Check sheet for the drawn part. Datum: minimum x, y, z corner. Units: mm. A direction names the side the tool comes from. Round coordinates to 2 decimals unless told otherwise and drop trailing zeros. Write each loop counter-clockwise with the first axis right and the second up, starting at its lowest first coordinate (ties: lowest second). Pieces come first, ordered by that corner, then holes. Notation, with made-up numbers: (65, -11) - (113, -11) arc R21 ccw to (113, 18) - close; hole circle Ø6 at (1, 84.25). An arc over 180 degrees is marked (long way). Answer as a JSON object with one key per item and string values.
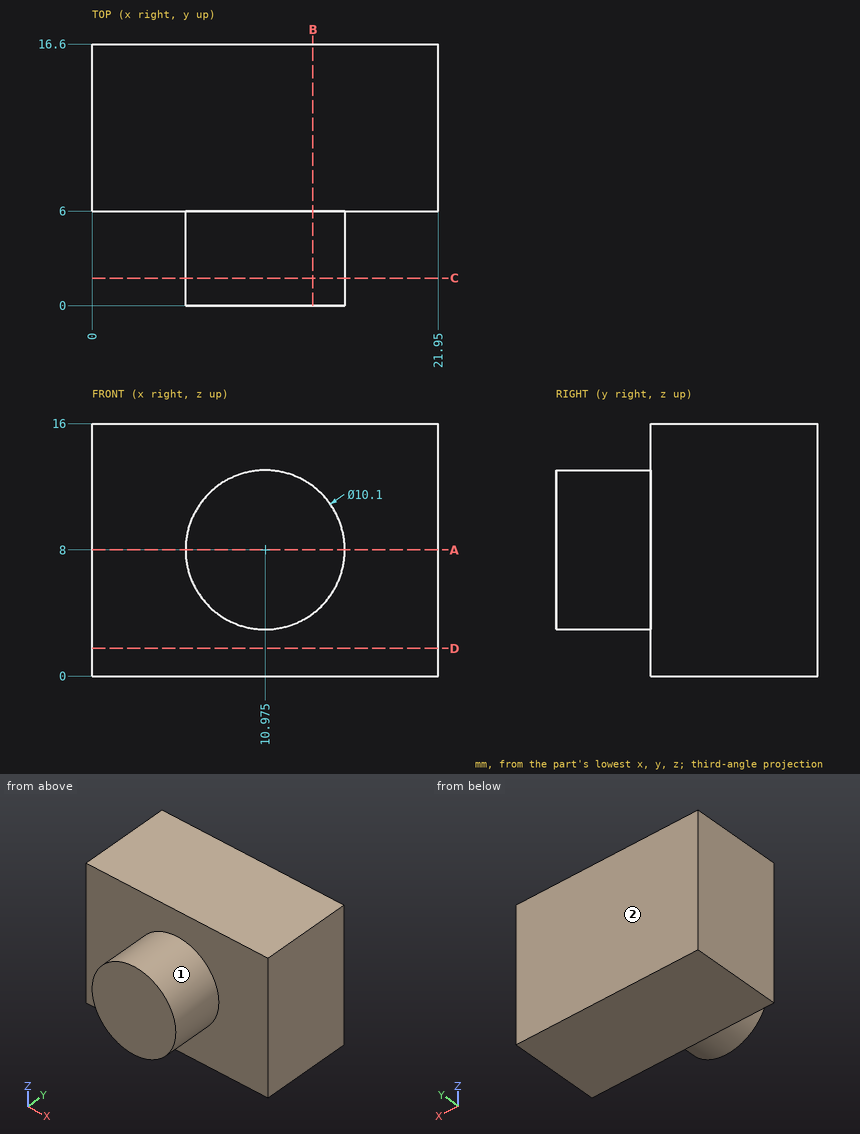
Q1. Section check D-D, the plane z = 1.75. Record the cut outline in (x, y).
Geometry check:
{"outline": "(0, 6) - (21.95, 6) - (21.95, 16.6) - (0, 16.6) - close"}
Q2. Set-up check for the marked faces 1 and 2: record each of +Z, -Z, +X, -X, +Y, -Y from which the full face is reachable in a straight line by a thin tool's end or side.
Geometry check:
{"face 1": "-Y", "face 2": "+Z, -Z, +X, -X, +Y"}
Q3. Section check B-B, the plane x = 14. Record the cut outline in (y, z).
Geometry check:
{"outline": "(0, 3.96) - (6, 3.96) - (6, 0) - (16.6, 0) - (16.6, 16) - (6, 16) - (6, 12.04) - (0, 12.04) - close"}
Q4. Section check C-C, the plane y = 1.75. Record the cut outline in (x, z) (3 decimals).
Geometry check:
{"outline": "circle Ø10.1 at (10.975, 8)"}
Q5. Section check A-A, the plane z = 8. Record the cut outline in (x, y) (3 decimals).
Geometry check:
{"outline": "(0, 6) - (5.925, 6) - (5.925, 0) - (16.025, 0) - (16.025, 6) - (21.95, 6) - (21.95, 16.6) - (0, 16.6) - close"}
Q6. Material ranges on line 1 along Y through (x, z) = (4, 4.25); line 2 along Z through (x, y) = (15.5, 4); line 3 along Z through (x, y) = (14.25, 3), recorded low to high. Write a range as [from, to].
Geometry check:
{"line 1": "y = [6, 16.6]", "line 2": "z = [5.76, 10.24]", "line 3": "z = [4.16, 11.84]"}
